Answer from the drawing. Dimensions are ordinates in mm from the lowest x, y and z of the part. A direction names the side the tool comes from. Coordinates: 2 decimals unless noted, no trailing zeros. Order: outer loops, then holes, each group sorted by start corner. A loop starts at its lowest first (then second) coordinate and runs counter-clockwise, first axis right, second up. Notation, with made-up numbers: (8.5, 20.25) -> (61.5, 20.25) arc R18 ccw to (61.5, 34.25) -> close; hole circle Ø4 at (49.25, -6.5). An arc over 180 degrees is marked (long way). Answer in a Markdown table with one row per item.
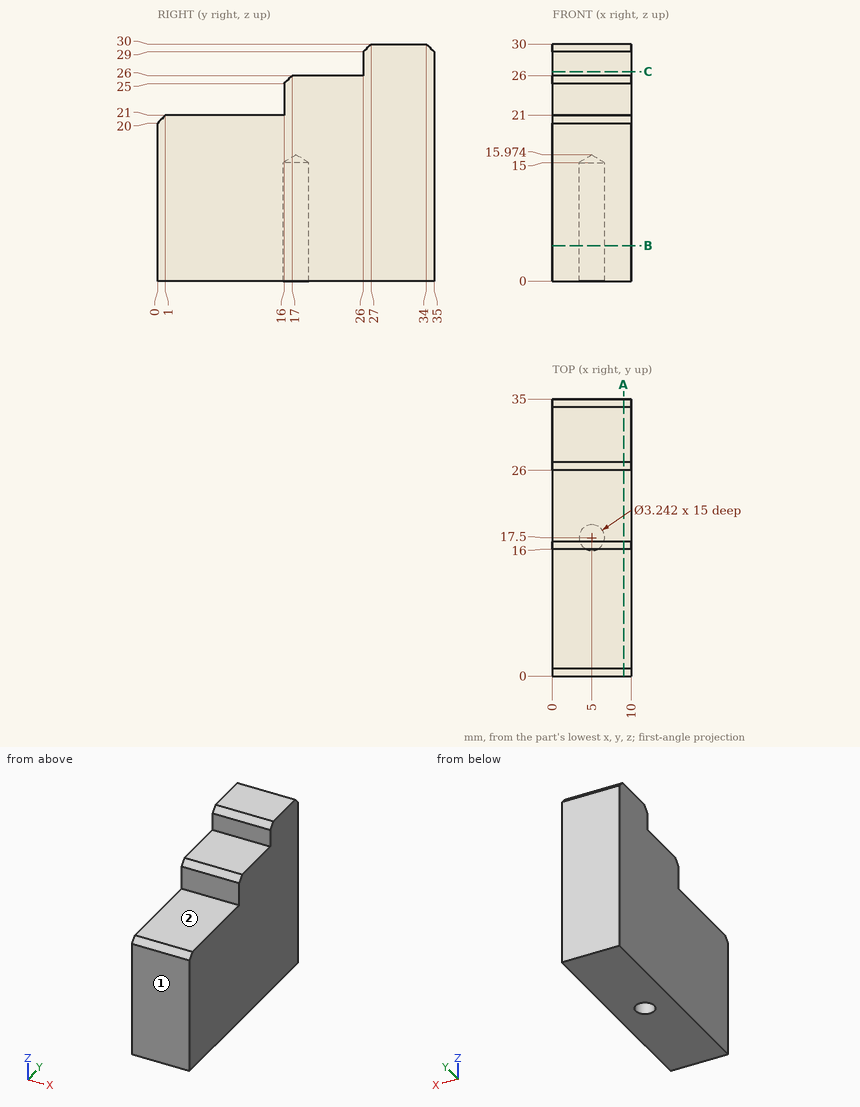
(1) A cutting plane is placed at B-B, the plane z = 4.5. Determine the outline of the cut face in (x, y).
Check values:
| item | result |
|---|---|
| outline | (0, 0) -> (10, 0) -> (10, 35) -> (0, 35) -> close; hole circle Ø3.24 at (5, 17.5) |
(2) A cutting plane is placed at C-C, the plane z = 26.5. Determine the outline of the cut face in (x, y), then the cut area to 3 significant figures.
Check values:
| item | result |
|---|---|
| outline | (0, 26) -> (10, 26) -> (10, 35) -> (0, 35) -> close |
| area | 90.0 mm² |
(3) A cutting plane is placed at A-A, the plane x = 9. Determine the outline of the cut face in (y, z), then the cut area to 3 significant figures.
Check values:
| item | result |
|---|---|
| outline | (0, 0) -> (35, 0) -> (35, 29) -> (34, 30) -> (27, 30) -> (26, 29) -> (26, 26) -> (17, 26) -> (16, 25) -> (16, 21) -> (1, 21) -> (0, 20) -> close |
| area | 864 mm² |
(4) Flat-ended cylindrical pins translate along their axes: pin 1 (1.2 mm diameter, centred on x = 4.5, z = 24, fed in from -Y); pin 2 (1.5 mm diameter, centred on x = 3.5, z = 27.5, fed in from -Y); pin 3 (1 mm diameter, centred on x = 2.5, y = 5.5, fed in from +Z). Find the tip coordinate at first contact, or state that the pin passes through.
Check values:
| item | result |
|---|---|
| pin 1 | y = 16 |
| pin 2 | y = 26 |
| pin 3 | z = 21 |
(5) Find the intervals of material crossed by line 1 along Y through (x, z) = (5, 4); line 2 along X through (y, z) = (17.5, 10.75); line 3 along Z through (x, y) = (5.5, 4), in increasing order. Write a range as from..to.
Check values:
| item | result |
|---|---|
| line 1 | 0..15.88, 19.12..35 |
| line 2 | 0..3.38, 6.62..10 |
| line 3 | 0..21 |
(6) Which of the six approach directions +Z, -Z, +X, -X, +Y, -Y give full straight-line access (tool end or side, diameter ignored) to the marked faces 1 and 2?
Check values:
| item | result |
|---|---|
| face 1 | +Z, -Z, +X, -X, -Y |
| face 2 | +Z, +X, -X, -Y |
